from build123d import *

# Parameters (mm, degrees)
BOSS_EXTRU_1_DEPTH = 47.3
BOSS_EXTRU_2_DEPTH = 12.7


with BuildPart() as part:
    # Esquisse1 → Boss.-Extru.1 (new body)
    with BuildSketch(Plane.XY):
        with BuildLine():
            Line((-95, -31.75), (95, -31.75))
            ThreePointArc((95, -31.75), (107.515790027, -26.565790027), (112.7, -14.05))
            Line((112.7, -14.05), (112.7, 14.05))
            ThreePointArc((112.7, 14.05), (107.515790027, 26.565790027), (95, 31.75))
            Line((95, 31.75), (-95, 31.75))
            ThreePointArc((-95, 31.75), (-107.515790027, 26.565790027), (-112.7, 14.05))
            Line((-112.7, 14.05), (-112.7, -14.05))
            ThreePointArc((-112.7, -14.05), (-107.515790027, -26.565790027), (-95, -31.75))
        make_face()
        with BuildLine():
            Line((-95, -19.05), (95, -19.05))
            ThreePointArc((95, -19.05), (98.535533906, -17.585533906), (100, -14.05))
            Line((100, -14.05), (100, 14.05))
            ThreePointArc((100, 14.05), (98.535533906, 17.585533906), (95, 19.05))
            Line((95, 19.05), (-95, 19.05))
            ThreePointArc((-95, 19.05), (-98.535533906, 17.585533906), (-100, 14.05))
            Line((-100, 14.05), (-100, -14.05))
            ThreePointArc((-100, -14.05), (-98.535533906, -17.585533906), (-95, -19.05))
        make_face(mode=Mode.SUBTRACT)
    extrude(amount=BOSS_EXTRU_1_DEPTH)

    # Esquisse2 → Boss.-Extru.2 (add)
    with BuildSketch(Plane.XY.offset(47.3)):
        with BuildLine():
            Line((-104.5, 14.05), (-104.5, -14.05))
            ThreePointArc((-104.5, -14.05), (-101.717514421, -20.767514421), (-95, -23.55))
            Line((-95, -23.55), (95, -23.55))
            ThreePointArc((95, -23.55), (101.717514421, -20.767514421), (104.5, -14.05))
            Line((104.5, -14.05), (104.5, 14.05))
            ThreePointArc((104.5, 14.05), (101.717514421, 20.767514421), (95, 23.55))
            Line((95, 23.55), (-95, 23.55))
            ThreePointArc((-95, 23.55), (-101.717514421, 20.767514421), (-104.5, 14.05))
        make_face()
        with BuildLine():
            Line((100, -14.05), (100, 14.05))
            ThreePointArc((100, 14.05), (98.535533906, 17.585533906), (95, 19.05))
            Line((95, 19.05), (-95, 19.05))
            ThreePointArc((-95, 19.05), (-98.535533906, 17.585533906), (-100, 14.05))
            Line((-100, 14.05), (-100, -14.05))
            ThreePointArc((-100, -14.05), (-98.535533906, -17.585533906), (-95, -19.05))
            Line((-95, -19.05), (95, -19.05))
            ThreePointArc((95, -19.05), (98.535533906, -17.585533906), (100, -14.05))
        make_face(mode=Mode.SUBTRACT)
    extrude(amount=BOSS_EXTRU_2_DEPTH)


solid = part.part
Check sheet for the modelled part. Datum: model origin and axes. Units: mm. A direction names the side the tool comes from. Round coordinates to 2 decimals unless told otherwise and drop trailing zeros. Write each loop counter-clockwise with the first axis right and the second up, starting at its lowest first coordinate (ties: lowest second). Pieces come first, ordered by that corner, then holes. Notation, with made-up numbers: (61, -3) -> (100, -3) arc R25 ccw to (100, 29) -> close; hole circle Ø8 at (4.25, 41). An arc over 180 degrees is marked (long way). Answer as CSV lines item,"result". Start each with the question number.
1) Tool access check on faces 1 (the flat face through (-100, 0, 30)), 2 (the cylindrical face through (-101.643, 20.841, 53.561)), 3 (the flat face through (-104.5, 0, 54)). Record the directions out of +Z, -Z, +X, -X, +Y, -Y that give a thin tool (end or side, any length) a straight path to the whole face; none if there is none.
2) Go/stop test with flat-tipped pins: P1, Ø6, axis at x = -41.5, y = -21, coming from the -Z side; P2, Ø10, axis at x = 20, z = 56, coming from the -Y side; P3, Ø4, axis at y = 1, z = 52.5, coming from the -X side; P4, Ø4, axis at y = 2, z = 51, coming from the +X side. Record where each tip stops, or that it passes through.
3) Section check B-B on z = 49.5. Enter the section's corners in (x, y).
4) Material ranges on line 1 (Y direction, x = -84.5, z = 46.5); line 2 (X direction, y = 11, z = 10); line 3 (Y direction, x = -78, z = 47.5), recorded low to high. Write a range as from..to.
5) Section check D-D on z = 19.5. Enter the section's corners in (x, y), and give its area (3 significant figures).
6) Section check C-C on x = -36. Enter the section's corners in (y, z).
7) Release check for a two-part mould opening along X. For faces 4 (the cylindrical face through (98.57, 17.55, 29.58)), 5 (the flat face through (104.5, 0, 54)), 6 (the flat face through (-1, -23.55, 54)) record: pulls with the +X half, pulls with the -X half, needs draft (parallel to the pull), parting line crosses it, or undercut.
8) Section check A-A on y = 7.5. Enter the section's corners in (x, z).
Found:
1,face 1,"+Z, -Z"
1,face 2,"+Z, -X, +Y"
1,face 3,"+Z, -X, +Y, -Y"
2,P1,"stops at z = 0"
2,P2,"stops at y = -23.55"
2,P3,"stops at x = -104.5"
2,P4,"stops at x = 104.5"
3,outline,"(-104.5, -14.05) arc R9.5 ccw to (-95, -23.55) -> (95, -23.55) arc R9.5 ccw to (104.5, -14.05) -> (104.5, 14.05) arc R9.5 ccw to (95, 23.55) -> (-95, 23.55) arc R9.5 ccw to (-104.5, 14.05) -> close; hole (-100, -14.05) arc R5 ccw to (-95, -19.05) -> (95, -19.05) arc R5 ccw to (100, -14.05) -> (100, 14.05) arc R5 ccw to (95, 19.05) -> (-95, 19.05) arc R5 ccw to (-100, 14.05) -> close"
4,line 1,"y = -31.75..-19.05, 19.05..31.75"
4,line 2,"x = -112.7..-100, 100..112.7"
4,line 3,"y = -23.55..-19.05, 19.05..23.55"
5,outline,"(-112.7, -14.05) arc R17.7 ccw to (-95, -31.75) -> (95, -31.75) arc R17.7 ccw to (112.7, -14.05) -> (112.7, 14.05) arc R17.7 ccw to (95, 31.75) -> (-95, 31.75) arc R17.7 ccw to (-112.7, 14.05) -> close; hole (-100, -14.05) arc R5 ccw to (-95, -19.05) -> (95, -19.05) arc R5 ccw to (100, -14.05) -> (100, 14.05) arc R5 ccw to (95, 19.05) -> (-95, 19.05) arc R5 ccw to (-100, 14.05) -> close"
5,area,"6,450 mm^2"
6,outline,"(-31.75, 0) -> (-19.05, 0) -> (-19.05, 60) -> (-23.55, 60) -> (-23.55, 47.3) -> (-31.75, 47.3) -> close; (19.05, 0) -> (31.75, 0) -> (31.75, 47.3) -> (23.55, 47.3) -> (23.55, 60) -> (19.05, 60) -> close"
7,face 4,"undercut"
7,face 5,"pulls with the +X half"
7,face 6,"needs draft"
8,outline,"(-112.7, 0) -> (-100, 0) -> (-100, 60) -> (-104.5, 60) -> (-104.5, 47.3) -> (-112.7, 47.3) -> close; (100, 0) -> (112.7, 0) -> (112.7, 47.3) -> (104.5, 47.3) -> (104.5, 60) -> (100, 60) -> close"
